```python
from build123d import *

# Parameters (mm, degrees)
SKETCH1_W           = 100
SKETCH1_H           = 100
BOSS_EXTRUDE1_DEPTH = 4
SKETCH2_R           = 4.7625
CUT_EXTRUDE1_DEPTH  = 71.823724839
SKETCH3_W           = 8.5
SKETCH3_H           = 8.5
CUT_EXTRUDE2_DEPTH  = 71.823724839
BOSS_EXTRUDE3_DEPTH = 29
BOSS_EXTRUDE4_DEPTH = 29
CUT_EXTRUDE4_DEPTH  = 77.426435217
BOSS_EXTRUDE5_DEPTH = 29
BOSS_EXTRUDE6_DEPTH = 29
SKETCH12_R          = 1.5
CUT_EXTRUDE5_DEPTH  = 79.0320447
CUT_EXTRUDE6_DEPTH  = 3
SKETCH15_R          = 1.5
CUT_EXTRUDE7_DEPTH  = 10
BOSS_EXTRUDE7_DEPTH = 33
SCALE1_SCALE        = 0.95


with BuildPart() as part:
    # Sketch1 → Boss-Extrude1 (new body)
    with BuildSketch(Plane(origin=(0, 0, 0), x_dir=(1, 0, 0), z_dir=(0, 1, 0))):
        Rectangle(SKETCH1_W, SKETCH1_H)
    extrude(amount=BOSS_EXTRUDE1_DEPTH)

    # Sketch2 → Cut-Extrude1 (cut, through all)
    with BuildSketch(Plane(origin=(0, 4, 0), x_dir=(1, 0, 0), z_dir=(0, 1, 0))):
        with Locations(Location((0, 0, 0), (0, 0, 270))):
            Circle(SKETCH2_R)
    extrude(amount=-CUT_EXTRUDE1_DEPTH, mode=Mode.SUBTRACT)

    # Sketch3 → Cut-Extrude2 (cut, through all)
    with BuildSketch(Plane(origin=(0, 4, 0), x_dir=(1, 0, 0), z_dir=(0, 1, 0))):
        with Locations((-45.75, 45.75)):
            Rectangle(SKETCH3_W, SKETCH3_H)
        with Locations((45.75, 45.75)):
            Rectangle(SKETCH3_W, SKETCH3_H)
        with Locations((45.75, -45.75)):
            Rectangle(SKETCH3_W, SKETCH3_H)
        with Locations((-45.75, -45.75)):
            Rectangle(SKETCH3_W, SKETCH3_H)
    extrude(amount=-CUT_EXTRUDE2_DEPTH, mode=Mode.SUBTRACT)

    # Sketch4 → Boss-Extrude3 (add)
    with BuildSketch(Plane(origin=(0, 4, 0), x_dir=(1, 0, 0), z_dir=(0, 1, 0))):
        with BuildLine():
            Line((-10.927389365, -13.022755533), (-11.891570779, -14.171822198))
            ThreePointArc((-11.891570779, -14.171822198), (0, -18.5), (11.891570779, -14.171822198))
            Line((11.891570779, -14.171822198), (10.927389365, -13.022755533))
            ThreePointArc((10.927389365, -13.022755533), (0, -17), (-10.927389365, -13.022755533))
        make_face()
        with BuildLine():
            Line((-13.022755533, -10.927389365), (-14.171822198, -11.891570779))
            ThreePointArc((-14.171822198, -11.891570779), (-18.5, 0), (-14.171822198, 11.891570779))
            Line((-14.171822198, 11.891570779), (-13.022755533, 10.927389365))
            ThreePointArc((-13.022755533, 10.927389365), (-17, 0), (-13.022755533, -10.927389365))
        make_face()
        with BuildLine():
            Line((-10.927389365, 13.022755533), (-11.891570779, 14.171822198))
            ThreePointArc((-11.891570779, 14.171822198), (0, 18.5), (11.891570779, 14.171822198))
            Line((11.891570779, 14.171822198), (10.927389365, 13.022755533))
            ThreePointArc((10.927389365, 13.022755533), (0, 17), (-10.927389365, 13.022755533))
        make_face()
        with BuildLine():
            Line((13.022755533, 10.927389365), (14.171822198, 11.891570779))
            ThreePointArc((14.171822198, 11.891570779), (18.5, 0), (14.171822198, -11.891570779))
            Line((14.171822198, -11.891570779), (13.022755533, -10.927389365))
            ThreePointArc((13.022755533, -10.927389365), (17, 0), (13.022755533, 10.927389365))
        make_face()
    extrude(amount=BOSS_EXTRUDE3_DEPTH)

    # Sketch7 → Boss-Extrude4 (add)
    with BuildSketch(Plane(origin=(0, 4, 0), x_dir=(1, 0, 0), z_dir=(0, 1, 0))):
        Polygon((-41.5, -41.5), (-41.5, -50), (-40, -50), (-40, -40), (-50, -40), (-50, -41.5), align=None)
        Polygon((40, -50), (40, -40), (50, -40), (50, -41.5), (41.5, -41.5), (41.5, -50), align=None)
        Polygon((50, 41.5), (50, 40), (40, 40), (40, 50), (41.5, 50), (41.5, 41.5), align=None)
        Polygon((-50, 41.5), (-50, 40), (-40, 40), (-40, 50), (-41.5, 50), (-41.5, 41.5), align=None)
    extrude(amount=BOSS_EXTRUDE4_DEPTH)

    # Sketch8 → Cut-Extrude4 (cut, through all)
    with BuildSketch(Plane(origin=(0, 4, 0), x_dir=(1, 0, 0), z_dir=(0, 1, 0))):
        Polygon((-14.171822198, -11.891570779), (-40, -50), (-36.17429682, -50), (-11.891570779, -14.171822198), (-9.867198001, -11.184942236), (-12.488706492, -9.408201793), align=None)
        Polygon((-11.891570779, 14.171822198), (-50, 40), (-50, 36.17429682), (-14.171822198, 11.891570779), (-11.184942236, 9.867198001), (-9.408201793, 12.488706492), align=None)
        Polygon((14.171822198, 11.891570779), (40, 50), (36.17429682, 50), (11.891570779, 14.171822198), (9.867198001, 11.184942236), (12.488706492, 9.408201793), align=None)
        Polygon((11.891570779, -14.171822198), (50, -40), (50, -36.17429682), (14.171822198, -11.891570779), (11.184942236, -9.867198001), (9.408201793, -12.488706492), align=None)
    extrude(amount=CUT_EXTRUDE4_DEPTH, mode=Mode.SUBTRACT)

    # Sketch9 → Boss-Extrude5 (add)
    with BuildSketch(Plane(origin=(0, 4, 0), x_dir=(1, 0, 0), z_dir=(0, 1, 0))):
        Polygon((-11.891570779, -14.171822198), (-36.17429682, -50), (-34.17429682, -50), (-10.52109933, -15.100666052), align=None)
        Polygon((-14.171822198, -11.891570779), (-40, -50), (-40, -47.049081084), (-14.981255079, -10.134937263), (-13.610783629, -11.063781117), align=None)
        Polygon((-50, 34.17429682), (-15.100666052, 10.52109933), (-14.171822198, 11.891570779), (-50, 36.17429682), align=None)
        Polygon((-11.891570779, 14.171822198), (-50, 40), (-47.049081084, 40), (-10.134937263, 14.981255079), (-11.063781117, 13.610783629), align=None)
        Polygon((34.17429682, 50), (10.52109933, 15.100666052), (11.891570779, 14.171822198), (36.17429682, 50), align=None)
        Polygon((14.171822198, 11.891570779), (40, 50), (40, 47.049081084), (14.981255079, 10.134937263), (13.610783629, 11.063781117), align=None)
        Polygon((50, -34.17429682), (15.100666052, -10.52109933), (14.171822198, -11.891570779), (50, -36.17429682), align=None)
        Polygon((11.891570779, -14.171822198), (50, -40), (47.049081084, -40), (10.134937263, -14.981255079), (11.063781117, -13.610783629), align=None)
    extrude(amount=BOSS_EXTRUDE5_DEPTH)

    # Sketch11 → Boss-Extrude6 (add)
    with BuildSketch(Plane(origin=(0, 4, 0), x_dir=(1, 0, 0), z_dir=(0, 1, 0))):
        Polygon((-40, -40), (-35.222450169, -40), (-40, -47.049081084), align=None)
        Polygon((-40, 40), (-40, 35.222450169), (-47.049081084, 40), align=None)
        Polygon((40, 40), (35.222450169, 40), (40, 47.049081084), align=None)
        Polygon((40, -40), (40, -35.222450169), (47.049081084, -40), align=None)
    extrude(amount=BOSS_EXTRUDE6_DEPTH)

    # Sketch12 → Cut-Extrude5 (cut, through all)
    with BuildSketch(Plane(origin=(0, 0, 0), x_dir=(-1, 0, 0), z_dir=(0, -1, 0))):
        with Locations(Location((-3.5, 33, 0), (0, 0, 90))):
            Circle(SKETCH12_R)
        with Locations(Location((-3.5, -33, 0), (0, 0, 90))):
            Circle(SKETCH12_R)
        with Locations(Location((-35, 33, 0), (0, 0, 90))):
            Circle(SKETCH12_R)
        with Locations(Location((-28, -33, 0), (0, 0, 90))):
            Circle(SKETCH12_R)
    extrude(amount=-CUT_EXTRUDE5_DEPTH, mode=Mode.SUBTRACT)

    # Sketch14 → Cut-Extrude6 (cut)
    with BuildSketch(Plane(origin=(0, 4, 0), x_dir=(1, 0, 0), z_dir=(0, 1, 0))):
        Polygon((28, -29.882308546), (25.3, -31.441154273), (25.3, -34.558845727), (28, -36.117691454), (30.7, -34.558845727), (30.7, -31.441154273), align=None)
        Polygon((3.5, -29.882308546), (0.8, -31.441154273), (0.8, -34.558845727), (3.5, -36.117691454), (6.2, -34.558845727), (6.2, -31.441154273), align=None)
        Polygon((3.5, 36.117691454), (0.8, 34.558845727), (0.8, 31.441154273), (3.5, 29.882308546), (6.2, 31.441154273), (6.2, 34.558845727), align=None)
        Polygon((35, 36.117691454), (32.3, 34.558845727), (32.3, 31.441154273), (35, 29.882308546), (37.7, 31.441154273), (37.7, 34.558845727), align=None)
    extrude(amount=-CUT_EXTRUDE6_DEPTH, mode=Mode.SUBTRACT)

    # Sketch15 → Cut-Extrude7 (cut)
    with BuildSketch(Plane(origin=(0, 33, 0), x_dir=(1, 0, 0), z_dir=(0, 1, 0))):
        with Locations(Location((44, -39, 0), (0, 0, 270))):
            Circle(SKETCH15_R)
        with Locations(Location((-39, -44, 0), (0, 0, 270))):
            Circle(SKETCH15_R)
        with Locations(Location((-44, 39, 0), (0, 0, 270))):
            Circle(SKETCH15_R)
        with Locations(Location((39, 44, 0), (0, 0, 270))):
            Circle(SKETCH15_R)
    extrude(amount=-CUT_EXTRUDE7_DEPTH, mode=Mode.SUBTRACT)

    # Sketch16 → Boss-Extrude7 (add)
    with BuildSketch(Plane.XZ):
        Polygon((-50, 41.5), (-50, 43.5), (-43.5, 43.5), (-43.5, 50), (-41.5, 50), (-41.5, 41.5), align=None)
        Polygon((50, 41.5), (41.5, 41.5), (41.5, 50), (43.5, 50), (43.5, 43.5), (50, 43.5), align=None)
        Polygon((50, -41.5), (50, -43.5), (43.5, -43.5), (43.5, -50), (41.5, -50), (41.5, -41.5), align=None)
        Polygon((-50, -41.5), (-41.5, -41.5), (-41.5, -50), (-43.5, -50), (-43.5, -43.5), (-50, -43.5), align=None)
    extrude(amount=-BOSS_EXTRUDE7_DEPTH)


with BuildPart() as part_1:
    # Scale1: scaled about (-0.08501153, 9.094594804, 0)
    add(part.part.scale(SCALE1_SCALE).moved(Location((-0.004250577, 0.45472974, 0))))


solid = part_1.part
```
Build history of the part. All positions in model axes, mm. A direction names the side the tool comes from. Coordinates: 2 decimals unless noted, no trailing zeros. Write each loop counter-clockwise with the first axis right and the second up, starting at its lowest first coordinate (ties: lowest second). Pieces come first, ordered by that corner, then holes.
1. Band-saw the part on B-B, the plane y = 19. Give the number of separate pieces and of enclosed holes in the cut face, and give its area (3 significant figures).
Answer block:
separate pieces: 4
enclosed holes: 0
area: 927 mm2
2. Drop flat-ended pins along their axis: pin 1 (12 mm diameter, centred on x = 0, z = 0, fed in from -Y); pin 2 (10 mm diameter, centred on x = 3.5, y = 19, fed in from -Z) (3 decimals); pin 3 (6 mm diameter, centred on x = 18, y = 8, fed in from +Z); pin 4 (1.4 mm diameter, centred on x = 41.5, z = 37.5, fed in from +Y). Give the stop position or say it passes through.
Answer block:
pin 1: stops at y = 0.45
pin 2: stops at z = -17.575
pin 3: stops at z = 21.94
pin 4: stops at y = 22.3
3. 3-axis set-ups, long thin cutter, end or side, ignore diameter. For faces 1 (the flat face through (2, 4.255, 34)), 2 (the flat face through (35.811, 3, -31)), 3 (the flat face through (-31.196, 17.837, -21.413)), 4 (the flat face through (31.188, 17.837, 21.413)): which of +Z, -Z, +X, -X, +Y, -Y reach the whole face in a straight line?
Answer block:
face 1: +Z, +Y
face 2: +Y
face 3: -X, +Y
face 4: +X, +Y
4. Drill centre lines: probe 1 along X at (y, z) = (1.15, -31.35); probe 2 along X at (y, z) = (1.2, 31.35); probe 3 along X at (y, z) = (13.5, -28). Where is each one in solid material? Low to high.
Answer block:
probe 1: x = -47.5 to 1.9, 4.75 to 31.82, 34.67 to 47.5
probe 2: x = -47.5 to 1.9, 4.75 to 25.17, 28.02 to 47.5
probe 3: x = -40.92 to -38.11, -32.75 to -29.95, 19.25 to 21.15, 24.78 to 26.68
5. Pull direction Z, two halves, no side cores. Call faces 5 (the flat face through (42, 22.305, 37)), 6 (the flat face through (-3, 4.255, -35)), 7 (the flat face through (3, 3, -47.5)), 8 (the cylindrical face through (41.25, 27.121, 38.366)): released by +Z, released by -Z, zero draft, split by the parting line, or undercut.
Answer block:
face 5: undercut
face 6: zero draft
face 7: released by -Z
face 8: undercut
6. Band-saw the part on A-A, the plane z = 0. Give the cut face in (x, y).
Answer block:
outline: (-47.5, 0.45) - (-4.53, 0.45) - (-4.53, 4.25) - (-16.15, 4.25) - (-16.15, 31.8) - (-17.58, 31.8) - (-17.58, 4.25) - (-47.5, 4.25) - close; (4.52, 0.45) - (47.5, 0.45) - (47.5, 4.25) - (17.57, 4.25) - (17.57, 31.8) - (16.15, 31.8) - (16.15, 4.25) - (4.52, 4.25) - close
